from build123d import *

# Parameters (mm, degrees)
F0_R     = 12.5
F1_DEPTH = 45
F3_W     = 45
F3_H     = 200
F4_DEPTH = 20
F6_W     = 50
F6_H     = 15
F7_DEPTH = 25
F8_R     = 5
F9_DEPTH = 185.001


with BuildPart() as f1:
    # F0 (on Front) → F1 (new body)
    with BuildSketch(Plane.XZ):
        Circle(F0_R)
    extrude(amount=F1_DEPTH)

    # F3 (on offset) → F4 (join)
    with BuildSketch(Plane.XZ.offset(20)):
        Rectangle(F3_W, F3_H)
    extrude(amount=-F4_DEPTH)

    # F6 (on offset) → F7 (join)
    with BuildSketch(Plane.XZ.offset(-25)):
        with Locations((0, 77.5)):
            Rectangle(F6_W, F6_H)
        with Locations((0, -77.5)):
            Rectangle(F6_W, F6_H)
    extrude(amount=F7_DEPTH)

    # F8 (on face) → F9 (cut, through all)
    with BuildSketch(Plane.XY.offset(85)):
        with Locations((15, 12.5)):
            Circle(F8_R)
        with Locations((-15, 12.5)):
            Circle(F8_R)
    extrude(amount=-F9_DEPTH, mode=Mode.SUBTRACT)


solid = f1.part
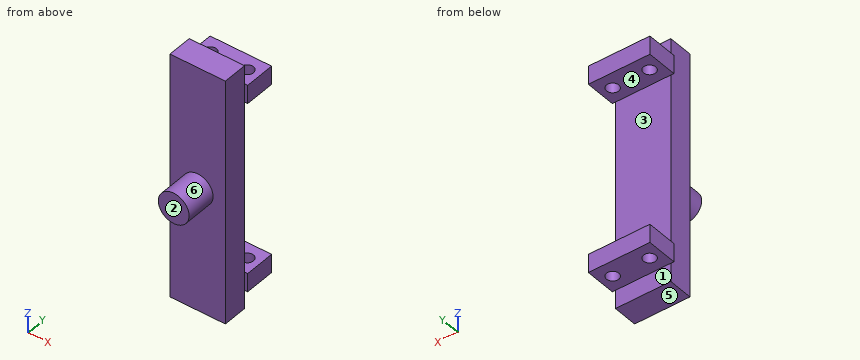
Can you work these out from the model? Positions are in its coordinate system, mm. Face numbers are marked on the shaded views. A direction names the side the tool comes from. Give positions to 0.01 mm unless a question says otherwise; leave off trailing zeros. Loops run counter-clockwise (first coordinate to the right, second up) from the corner with the lowest first, then second, coordinate; pieces in that order, holes last. Notation, with made-up numbers: (25.5, 59.25) -> (72.5, 59.25) arc R35 cw to (72.5, 96.25) -> close; hole circle Ø5 at (-9.5, 48.25). An arc over 180 degrees is marked (long way). Return JSON: item names as keys, results as strings.
Q1. I want a section at D-D, the plane y = 3.5. List the corners of the cut face in (x, z) for me, then the cut area to 3 significant figures.
Checks:
{"outline": "(-25, -85) -> (25, -85) -> (25, -70) -> (-25, -70) -> close; (-25, 70) -> (25, 70) -> (25, 85) -> (-25, 85) -> close", "area": "1,500 mm2"}
Q2. I want a section at C-C, the plane y = 12.5. List the corners of the cut face in (x, z) for me.
Checks:
{"outline": "(-25, -85) -> (-20, -85) -> (-20, -70) -> (-25, -70) -> close; (-25, 70) -> (-20, 70) -> (-20, 85) -> (-25, 85) -> close; (-10, -85) -> (10, -85) -> (10, -70) -> (-10, -70) -> close; (-10, 70) -> (10, 70) -> (10, 85) -> (-10, 85) -> close; (20, -85) -> (25, -85) -> (25, -70) -> (20, -70) -> close; (20, 70) -> (25, 70) -> (25, 85) -> (20, 85) -> close"}
Q3. On a 3-axis mill with a long thin cutter (end or side, diameter ignored), from which of +Z, -Z, +X, -X, +Y, -Y can I reach the whole of each face in a straight line? I mean the marked faces 1 and 2. Say none if no direction works.
Checks:
{"face 1": "-Z, +X, -X, +Y", "face 2": "+Z, -Z, +X, -X, -Y"}
Q4. We'd pull the mould along Z, two halves only. Please class the marked faces 3, 4, 5 and 6: released by +Z, released by -Z, zero draft, split by the parting line, or undercut.
Checks:
{"face 3": "undercut", "face 4": "undercut", "face 5": "released by -Z", "face 6": "split by the parting line"}
Q5. I want a section at B-B, the plane x = 15. List the corners of the cut face in (y, z) for me.
Checks:
{"outline": "(-20, -100) -> (0, -100) -> (0, -85) -> (7.5, -85) -> (7.5, -70) -> (0, -70) -> (0, 70) -> (7.5, 70) -> (7.5, 85) -> (0, 85) -> (0, 100) -> (-20, 100) -> close; (17.5, -85) -> (25, -85) -> (25, -70) -> (17.5, -70) -> close; (17.5, 70) -> (25, 70) -> (25, 85) -> (17.5, 85) -> close"}
Q6. I want a section at A-A, the plane z = -83. List the corners of the cut face in (x, y) for me.
Checks:
{"outline": "(-25, 0) -> (-22.5, 0) -> (-22.5, -20) -> (22.5, -20) -> (22.5, 0) -> (25, 0) -> (25, 25) -> (-25, 25) -> close; hole circle Ø10 at (-15, 12.5); hole circle Ø10 at (15, 12.5)"}
Q7. I need wall thicknesses on probe 1 along X at (y, z) = (12, -79); probe 2 along Y at (x, z) = (-15, -77.25); probe 3 along Z at (x, y) = (-14, 18). Which ranges of each line are inside material? Lowest first, please.
Checks:
{"probe 1": "x = -25 to -19.97, -10.03 to 10.03, 19.97 to 25", "probe 2": "y = -20 to 7.5, 17.5 to 25", "probe 3": "z = -85 to -70, 70 to 85"}
Q8. For pin 1 Ø6 at (x, y) = (15, 12.5) entering from +Z; pin 2 Ø12.5 at (x, y) = (-7.5, 18.5) entering from +Z; pin 3 Ø16 at (y, z) = (-6.5, -12.5) entering from +X; pin 4 Ø12 at (x, y) = (0, -37) entering from -Z, each with a flat end and sliding along its axis, tell me the tip position at first contact or that it passes through.
Checks:
{"pin 1": "passes through", "pin 2": "stops at z = 85", "pin 3": "stops at x = 22.5", "pin 4": "stops at z = -12.5"}
